Read the model definition and answer for the solid it produces. Units are mm, in the model's axes. Give positions to 0.01 mm unless a question says otherwise; leave off trailing zeros. Order: outer loops, then holes, each group sorted by start corner. A loop starts at its lowest first (then second) coordinate and runs counter-clockwise, first axis right, second up. Notation, with made-up numbers: M 26,53.5 L 52,53.5 A27 cw 52,90.5 Z; hole C -1,-16 d4. An arc over 180 degrees is marked long. Write item = value, one per line. Start each with the question number.
from build123d import *

# Parameters (mm, degrees)
F0_W     = 406.4
F0_H     = 304.8
F1_DEPTH = 4.7625
F2_R     = 12.192
F2_R_2   = 9.525
F2_W     = 10.16
F2_H     = 7.874
F2_R_3   = 12.7
F2_R_4   = 6.35
F2_R_5   = 3.175
F2_H_2   = 10.16
F3_DEPTH = 25.4
F4_R     = 9.525
F4_W     = 76.2
F4_H     = 19.05
F5_DEPTH = 25.4


with BuildPart() as f1:
    # F0 (on Top) → F1 (new body)
    with BuildSketch(Plane.XY):
        with Locations((-15.715082, 10.855626)):
            Rectangle(F0_W, F0_H)
    extrude(amount=F1_DEPTH)

    # F2 (on Top) → F3 (cut)
    with BuildSketch(Plane.XY):
        with Locations((-142.715082, 87.055626)):
            Circle(F2_R)
        with Locations((-142.715082, 10.855626)):
            Circle(F2_R_2)
        with Locations((-142.715082, -39.944374)):
            Circle(F2_R_2)
        with Locations((-15.715082, -39.944374)):
            Circle(F2_R_2)
        with Locations((-15.715082, 10.855626)):
            Circle(F2_R_2)
        with Locations((-160.495082, 159.318626)):
            Rectangle(F2_W, F2_H)
        with Locations((60.484918, 10.855626)):
            Circle(F2_R_2)
        with Locations((111.284918, 10.855626)):
            Circle(F2_R_2)
        with Locations((162.084918, 10.855626)):
            Circle(F2_R_2)
        with Locations((86.052007, 54.064918)):
            Circle(F2_R_3)
        with Locations((132.892046, 54.978594)):
            Circle(F2_R_3)
        with Locations((-79.215082, -7.533974)):
            Circle(F2_R_3)
        with Locations((149.384918, 150.555626)):
            Circle(F2_R_4)
        with Locations((-52.545082, 131.124626)):
            Circle(F2_R_5)
        with Locations((-103.345082, 131.124626)):
            Circle(F2_R_5)
        with Locations((-193.515082, 150.555626)):
            Rectangle(F2_W, F2_H_2)
        with Locations((-15.715082, 87.055626)):
            Circle(F2_R)
    extrude(amount=F3_DEPTH, mode=Mode.SUBTRACT)

    # F4 (on face) → F5 (cut)
    with BuildSketch(Plane.XY.offset(4.7625)):
        with Locations((-142.715082, -103.444374)):
            Circle(F4_R)
        with Locations((-100.297082, -103.444374)):
            Circle(F4_R)
        with Locations((73.184918, -65.344374)):
            Circle(F4_R)
        with Locations((73.184918, -116.144374)):
            Circle(F4_R)
        with Locations((123.984918, -65.344374)):
            Circle(F4_R)
        with Locations((123.984918, -116.144374)):
            Circle(F4_R)
        with Locations((-57.879082, -103.444374)):
            Circle(F4_R)
        with Locations((-15.461082, -103.444374)):
            Circle(F4_R)
        with Locations((-77.310082, 134.299626)):
            Rectangle(F4_W, F4_H)
    extrude(amount=-F5_DEPTH, mode=Mode.SUBTRACT)


solid = f1.part
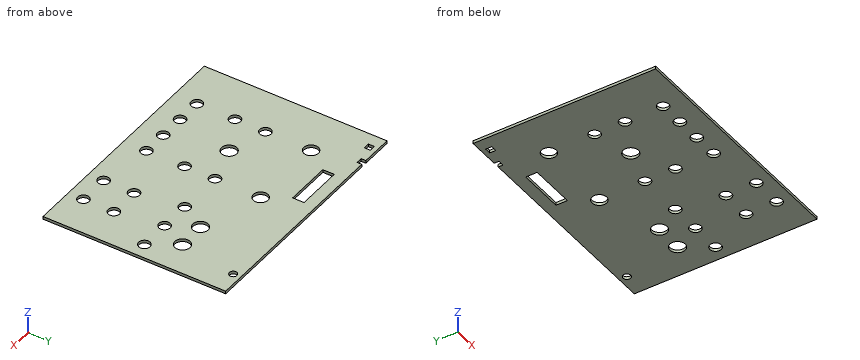
1) This flat-tipped pin is pushed along its axis until it touches: P1, Ø22, axis at x = 162.08, y = 10.86, coming from the -Z side. Where does it stop, or does it pass through?
2) Find the intervals of material crossed by probe 1 along Y at (x, z) = (-100.5, 1.75); probe 2 along Y at (x, z) = (76.5, 1.5); probe 3 along X at (y, z) = (-120.5, 1.95), in increasing order. Write a range as [from, to].
3) Find section B-B on x = -99.5. Determine the outline of the cut face in (y, z).
4) Find section D-D on z = 2.2. Count the separate pieces of the cut face and the enclosed holes in it, plus the area to 3 significant figures.
5) Find section A-A on y = -3. Determine the outline of the cut face in (x, z).
6) Find section C-C on y = 94. Determine the outline of the cut face in (x, z), plus the area to 3 significant figures.
Numbers:
q1.P1 = 0
q2.probe_1 = [-141.54, -112.97], [-93.92, 124.77], [143.82, 163.26]
q2.probe_2 = [-141.54, -125.07], [-107.21, -74.27], [-56.41, 45.7], [62.43, 163.26]
q2.probe_3 = [-218.92, 64.71], [81.66, 115.51], [132.46, 187.48]
q3.outline = M -141.54,0 L -112.94,0 L -112.94,4.76 L -141.54,4.76 Z; M -93.95,0 L 124.77,0 L 124.77,4.76 L -93.95,4.76 Z; M 143.82,0 L 163.26,0 L 163.26,4.76 L 143.82,4.76 Z
q4.separate_pieces = 1
q4.enclosed_holes = 23
q4.area = 115,000 mm2
q5.outline = M -218.92,0 L -91.08,0 L -91.08,4.76 L -218.92,4.76 Z; M -67.35,0 L 187.48,0 L 187.48,4.76 L -67.35,4.76 Z
q6.outline = M -218.92,0 L -152.74,0 L -152.74,4.76 L -218.92,4.76 Z; M -132.69,0 L -25.74,0 L -25.74,4.76 L -132.69,4.76 Z; M -5.69,0 L 187.48,0 L 187.48,4.76 L -5.69,4.76 Z
q6.area = 1,740 mm2
